Here's how the part is built. I have some questions about the finished solid (model axes, mm). Face numbers are marked on the shaded views. Round coordinates to 2 decimals unless told otherwise and drop trailing zeros. Loops run counter-clockwise (first coordinate to the right, second up) from the corner with the lowest first, then second, coordinate; pieces in that order, holes last. Notation, with made-up numbers: M 67.25,-2.75 L 94.25,-2.75 A19 ccw 94.25,25.25 Z; hole C 83.5,25 d8. An arc over 180 degrees is marked long. Answer as a JSON object with one key per item and string values.
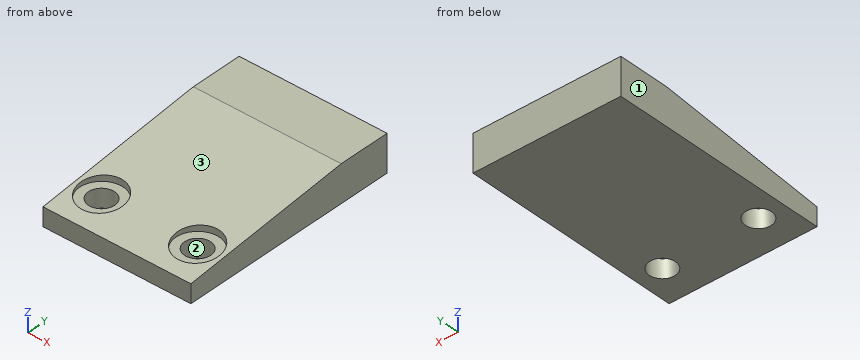
Autodesk Inventor part; units mm, degrees
ref_plane "Work Plane1" through (12.7, 14.605, 6.35) normal (0, 0, 1) x (1, 0, 0)
ref_plane "YZ Plane" through (0, 0, 0) normal (1, 0, 0) x (0, 1, 0)
ref_plane "XZ Plane" through (0, 0, 0) normal (0, 1, 0) x (-1, 0, 0)
sketch "Sketch1" plane through (0, 0, 0) normal (0, 0, 1) x (1, 0, 0)
  line L0 (12.7, -19.05) -> (-12.7, -19.05)
  line L1 (-12.7, -19.05) -> (-12.7, 19.05)
  line L2 (-12.7, 19.05) -> (12.7, 19.05)
  line L3 (12.7, 19.05) -> (12.7, -19.05)
  line L4 (12.7, -19.05) -> (-12.7, 19.05) construction
  line L5 (-12.7, -19.05) -> (12.7, 19.05) construction
  circle A0 centre (-8.255, -12.7) radius 2.25
  circle A1 centre (8.255, -12.7) radius 2.25
  line L6 (0, 19.05) -> (0, -19.05) construction
  line L7 (-6.005, 19.05) -> (-6.005, -19.05) construction
  line L8 (6.005, 19.05) -> (6.005, -19.05) construction
  line L9 (-6.005, 19.05) -> (2.4874, 19.05) construction
  circle A2 centre (-8.255, -12.7) radius 3.75
  circle A3 centre (8.255, -12.7) radius 3.75
  point P0 (0, 0)
  point P1 (0, 13.045)
  dimension "d0" = 25.4
  dimension "d1" = 38.1
  dimension "d2" = 4.5
  dimension "d3" = 4.5
  dimension "d4" = 8.255
  dimension "d5" = 8.255
  dimension "d6" = 6.35
  dimension "d7" = 6.35
  dimension "d14" = 7.5
  dimension "d15" = 7.5
extrude "Extrusion1" add sketch "Sketch1" along normal blind 6.35 contours L0 L1 L2 L3 | A2 | A3
sketch "Sketch2" plane through (12.7, -19.05, 0) normal (1, 0, 0) x (0, 0, -1)
  line L0 (-6.35, 32.095) -> (-6.35, 38.1)
  line L1 (0, 38.1) -> (0, 0)
  line L2 (-6.35, 38.1) -> (0, 38.1)
  line L3 (0, 38.1) -> (0, 29.21)
  line L4 (0, 29.21) -> (-6.35, 29.21)
  line L5 (-6.35, 29.21) -> (-6.35, 38.1)
  line L6 (-6.35, 29.21) -> (-3.175, 0)
  line L7 (0, 0) -> (-6.35, 0)
  line L8 (-3.175, 0) -> (0, 0)
  line L9 (-6.35, 4.1) -> (0, 4.1)
  line L10 (0, 0) -> (0, 38.1)
  line L11 (0, 38.1) -> (-6.35, 38.1)
  line L12 (-6.35, 0) -> (-6.35, 38.1)
  line L13 (0, 0) -> (-6.35, 0)
  point P0 (0, 19.05)
  dimension "d11" = 8.89
extrude "Extrusion2" cut sketch "Sketch2" against normal through all contours L6 L9 L12 | L6 L7 L12 L9
ref_plane "Work Plane1" through (12.7, 14.605, 6.35) normal (0, 0, 1) x (1, 0, 0)
sketch "Sketch3" plane through (12.7, 14.605, 6.35) normal (0, 0, 1) x (1, 0, 0)
  line L0 (-25.4, -33.655) -> (-25.4, -4.445)
  line L1 (0, -33.655) -> (-25.4, -33.655)
  line L2 (0, -4.445) -> (0, -33.655)
  line L3 (-25.4, -4.445) -> (0, -4.445)
  circle A0 centre (-4.445, -27.305) radius 2.25
  circle A1 centre (-20.955, -27.305) radius 2.25
  circle A2 centre (-20.955, -27.305) radius 2.25
  circle A3 centre (-20.955, -27.305) radius 3.75
  circle A4 centre (-4.445, -27.305) radius 3.75
  point P0 (-12.7, -14.605)
  dimension "d16" = 7.5
  dimension "d17" = 7.5
extrude "Extrusion3" cut sketch "Sketch3" against normal blind 3.175 contours A1 | A3 | A4
properties part number "Drone_Launcher_Stopper"
Item 1: We'd pull the mould along Y, two halves only. Please class the marked faces 1, 2 and 3: +Y half, -Y half, draft (parallel to the pull), parting line (faces both ways), or undercut.
Solution:
{"face 1": "draft", "face 2": "undercut", "face 3": "-Y half"}
Item 2: I want a section at B-B on y = -12.7. List the corners of the cut face in (x, z) for me (3 decimals), plus the area to 3 significant figures.
Solution:
{"outline": "M -12.7,0 L -10.505,0 L -10.505,3.175 L -12.005,3.175 L -12.005,3.865 L -12.7,3.865 Z; M -6.005,0 L 6.005,0 L 6.005,3.175 L 4.505,3.175 L 4.505,3.865 L -4.505,3.865 L -4.505,3.175 L -6.005,3.175 Z; M 10.505,0 L 12.7,0 L 12.7,3.865 L 12.005,3.865 L 12.005,3.175 L 10.505,3.175 Z", "area": "59.2 mm2"}
Item 3: For P1, Ø1, axis at x = -6, y = -2.5, coming from the +Z side; P2, Ø4, axis at x = 8.255, y = -12.7, coming from the -Z side; P3, Ø8.5, axis at x = -8.255, y = -12.7, coming from the +Z side; P4, Ø4, axis at x = 7, y = -12, coming from the +Z side (3 decimals), each with a flat end and sliding along its axis, tell me the tip position at first contact or that it passes through.
Solution:
{"P1": "stops at z = 5.03", "P2": "passes through", "P3": "stops at z = 4.33", "P4": "stops at z = 3.175"}
Item 4: If I drill on L1, parallel to X at y = -12.7, z = 3.45 (3 decimals); L2, parallel to X at y = -14, z = 2.5; L3, parallel to Y at x = 8.25, z = 2.75, over which ranges is the centre line in solid material (lowest first)? Write a range as from..to.
Solution:
{"L1": "x = -12.7..-12.005, -4.505..4.505, 12.005..12.7", "L2": "x = -12.7..-10.09, -6.42..6.42, 10.09..12.7", "L3": "y = -19.05..-14.95, -10.45..19.05"}
Item 5: I want a section at D-D on z = 5. List the corners of the cut face in (x, y) for me, plus the area to 3 significant figures.
Solution:
{"outline": "M -12.7,-2.26 L 12.7,-2.26 L 12.7,19.05 L -12.7,19.05 Z", "area": "541 mm2"}
Item 6: I want a section at C-C on x = 3.25. List the corners of the cut face in (y, z) for me (3 decimals).
Solution:
{"outline": "M -19.05,0 L 19.05,0 L 19.05,6.35 L 10.16,6.35 L -19.05,3.175 Z"}
